Study the drawing (mm; zero at the part's minimum x, y, z) and answer. A direction names the side the tool comes from. Round coordinates to 2 decimals unless told otherwise and drop trailing zeros. Write each loop counter-clockwise with the first axis right and the second up, starting at its lowest first coordinate (ties: lowest second). Pieces come first, ordered by that corner, then holes.
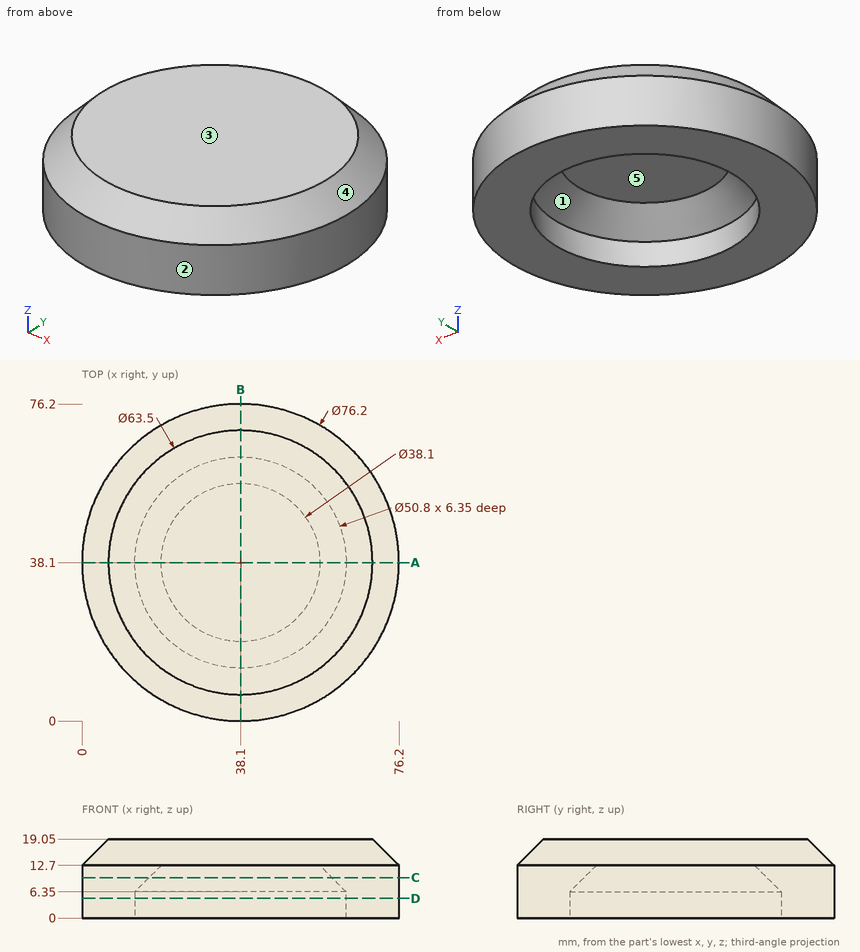
Q1. Given pin 1 (2 mm diameter, centred on x = 63.5, z = 16.5, fed in from +Y); pin 2 (8 mm diameter, centred on x = 50.5, z = 12, fed in from -Y); pin 3 (5 mm diameter, centred on y = 17.5, z = 16, fed in from +X), each flat-ended and moving along its own axis, determine where each tip first touches the part or whether it passes through.
Q2. Find the intervals of material crossed by L1, parallel to Y at x = 38.1, z = 1.5; L2, parallel to X at y = 42, z = 5.5; L3, parallel to Z at x = 51, y = 31.5, in increasing order.
Q3. Find section C-C (z = 9.75). Determine the outline of the cut face in (x, y).
Q4. The mould has two halves that part along X. Classify the marked faces 1, 2 and 3: +X half, -X half, draft (parallel to the pull), parting line (faces both ways), or undercut.
Q5. A tool of negligible diameter and unlimited length cuts with its end or side. For the marked faces 4 and 5, from which of +Z, -Z, +X, -X, +Y, -Y can it reach the whole face along a straight path? Write none if from no direction.
Q6. Find section A-A (y = 38.1). Determine the outline of the cut face in (x, z).
Q7. Find section D-D (z = 4.75). Determine the outline of the cut face in (x, y), plus the area to 3 significant figures.
Report:
1. pin 1: stops at y = 62.94
1. pin 2: stops at y = 0.94
1. pin 3: stops at x = 69.6
2. L1: y = 0 to 12.7, 63.5 to 76.2
2. L2: x = 0.2 to 13, 63.2 to 76
2. L3: z = 12.7 to 19.05
3. outline: circle Ø76.2 at (38.1, 38.1); hole circle Ø44 at (38.1, 38.1)
4. face 1: undercut
4. face 2: parting line
4. face 3: draft
5. face 4: +Z
5. face 5: -Z
6. outline: (0, 0) - (12.7, 0) - (12.7, 6.35) - (19.05, 12.7) - (57.15, 12.7) - (63.5, 6.35) - (63.5, 0) - (76.2, 0) - (76.2, 12.7) - (69.85, 19.05) - (6.35, 19.05) - (0, 12.7) - close
7. outline: circle Ø76.2 at (38.1, 38.1); hole circle Ø50.8 at (38.1, 38.1)
7. area: 2,530 mm2
